```python
from build123d import *

# Parameters (mm, degrees)
EXTRUDE002_DEPTH = 2.15
SKETCH002_W      = 82.25
SKETCH002_H      = 45.1
SKETCH002_R      = 1.65
EXTRUDE003_DEPTH = 1.6
SKETCH004_W      = 7
SKETCH004_H      = 24
EXTRUDE004_DEPTH = 8.5
SKETCH048_W      = 9
SKETCH048_H      = 4
SKETCH048_W_2    = 4
SKETCH048_H_2    = 7.5
EXTRUDE049_DEPTH = 8.5
SKETCH005_W      = 7
SKETCH005_H      = 37.5
EXTRUDE005_DEPTH = 8.5


with BuildPart() as obj1:
    # Sketch003 → Extrude002 (new body)
    with BuildSketch(Plane.XY):
        Polygon((76.75, 36.6), (76.75, 17.05), (59.85, 17.05), (59.85, 6.1), (8.6, 6.1), (8.6, 39.3), (16.6, 39.3), (16.6, 36.6), align=None)
    extrude(amount=-EXTRUDE002_DEPTH)


with BuildPart() as obj2:
    # Sketch002 → Extrude003 (new body)
    with BuildSketch(Plane.XY):
        with Locations((41.125, 22.55)):
            Rectangle(SKETCH002_W, SKETCH002_H)
        with Locations((3, 42.1)):
            Circle(SKETCH002_R, mode=Mode.SUBTRACT)
        with Locations((79.25, 42.1)):
            Circle(SKETCH002_R, mode=Mode.SUBTRACT)
        with Locations((3, 3)):
            Circle(SKETCH002_R, mode=Mode.SUBTRACT)
        with Locations((79.25, 3)):
            Circle(SKETCH002_R, mode=Mode.SUBTRACT)
    extrude(amount=EXTRUDE003_DEPTH)


with BuildPart() as obj3:
    # Sketch004 → Extrude004 (new body)
    with BuildSketch(Plane.XY):
        with Locations((74.85, 25.84)):
            Rectangle(SKETCH004_W, SKETCH004_H)
    extrude(amount=EXTRUDE004_DEPTH)


with BuildPart() as obj3_1:
    # Extrude004 placement: moved
    add(obj3.part.moved(Location((0, 0, 1.6))))


with BuildPart() as obj4:
    # Sketch048 → Extrude049 (new body)
    with BuildSketch(Plane.XY):
        with Locations((47.75, 36.6)):
            Rectangle(SKETCH048_W, SKETCH048_H)
        with Locations((36.25, 21.85)):
            Rectangle(SKETCH048_W_2, SKETCH048_H_2)
    extrude(amount=EXTRUDE049_DEPTH)


with BuildPart() as obj5:
    # Sketch005 → Extrude005 (new body)
    with BuildSketch(Plane.XY):
        with Locations((9.77, 21.95)):
            Rectangle(SKETCH005_W, SKETCH005_H)
    extrude(amount=EXTRUDE005_DEPTH)


with BuildPart() as obj5_1:
    # Extrude005 placement: moved
    add(obj5.part.moved(Location((0, 0, 1.6))))

    # Fusion001: union obj1, obj2, obj3, obj4
    add(obj1.part)
    add(obj2.part)
    add(obj3_1.part)
    add(obj4.part)


with BuildPart() as obj5_2:
    # Fusion001 placement: moved
    add(obj5_1.part.moved(Location((0, 0, 4))))


solid = obj5_2.part
```
The listing builds one solid part. Answer for the finished solid, in the listing's coordinates (mm). A direction names the side the tool comes from. Coordinates: 2 decimals unless noted, no trailing zeros. Loops run counter-clockwise (first coordinate to the right, second up) from the corner with the lowest first, then second, coordinate; pieces in that order, holes last. Notation, with made-up numbers: (46, 9.25) - (66, 9.25) arc R25 cw to (66, 41.25) - close; hole circle Ø8 at (-15.75, 54.5). An arc over 180 degrees is marked (long way). Use a Markdown table: item, result. Add a question column.
1) The part is cut by section B-B, the plane y = 42.1. Give the vertices of the cut face in (x, z).
2) The part is cut by section D-D, the plane y = 11. Give the vertices of the cut face in (x, z), and give its area (3 significant figures).
3) The part is cut by section C-C, the plane z = 10.25. Give the vertices of the cut face in (x, y), and give its area (4 significant figures).
4) For faces 1 (the flat face through (75, 13.84, 10)), 2 (the flat face through (71.35, 26, 10)), 3 (the flat face through (8.6, 22, 3)), determine the directions among +Z, -Z, +X, -X, +Y, -Y from which every point of the face is accessible in a straight line to the end or side of a thin tool.
5) Given pin 1 (3.5 mm diameter, centred on x = 74.5, z = 9, fed in from +Y); pin 2 (2.5 mm diameter, centred on y = 20.5, z = 11, fed in from -X); pin 3 (2.5 mm diameter, centred on x = 79.25, y = 42.1, fed in from -Z); pin 4 (1.7 mm diameter, centred on x = 12, z = 2.5, fed in from +Y), each flat-ended and moving along its own axis, determine where each tip first touches the part or whether it passes through.
6) Find the intervals of material crossed by line 1 (X direction, y = 23, z = 8.25); line 2 (Y direction, x = 79.25, z = 4.55); line 3 (X direction, y = 28.5, z = 8), in increasing order.
7) The part is cut by section A-A, the plane x = 79.25. Give the vertices of the cut face in (y, z), and give its area (3 significant figures).
Here are the results:
| question | item | result |
|---|---|---|
| 1 | outline | (0, 4) - (1.35, 4) - (1.35, 5.6) - (0, 5.6) - close; (4.65, 4) - (77.6, 4) - (77.6, 5.6) - (4.65, 5.6) - close; (80.9, 4) - (82.25, 4) - (82.25, 5.6) - (80.9, 5.6) - close |
| 2 | outline | (0, 4) - (8.6, 4) - (8.6, 1.85) - (59.85, 1.85) - (59.85, 4) - (82.25, 4) - (82.25, 5.6) - (13.27, 5.6) - (13.27, 14.1) - (6.27, 14.1) - (6.27, 5.6) - (0, 5.6) - close |
| 2 | area | 301 mm^2 |
| 3 | outline | (6.27, 3.2) - (13.27, 3.2) - (13.27, 40.7) - (6.27, 40.7) - close; (34.25, 18.1) - (38.25, 18.1) - (38.25, 25.6) - (34.25, 25.6) - close; (43.25, 34.6) - (52.25, 34.6) - (52.25, 38.6) - (43.25, 38.6) - close; (71.35, 13.84) - (78.35, 13.84) - (78.35, 37.84) - (71.35, 37.84) - close |
| 3 | area | 496.5 mm^2 |
| 4 | face 1 | +Z, +X, -Y |
| 4 | face 2 | +Z, +Y, -Y |
| 4 | face 3 | -Z, -X, +Y, -Y |
| 5 | pin 1 | stops at y = 37.84 |
| 5 | pin 2 | stops at x = 6.27 |
| 5 | pin 3 | passes through |
| 5 | pin 4 | stops at y = 39.3 |
| 6 | line 1 | x = 6.27 to 13.27, 34.25 to 38.25, 71.35 to 78.35 |
| 6 | line 2 | y = 0 to 1.35, 4.65 to 40.45, 43.75 to 45.1 |
| 6 | line 3 | x = 6.27 to 13.27, 71.35 to 78.35 |
| 7 | outline | (0, 4) - (1.35, 4) - (1.35, 5.6) - (0, 5.6) - close; (4.65, 4) - (40.45, 4) - (40.45, 5.6) - (4.65, 5.6) - close; (43.75, 4) - (45.1, 4) - (45.1, 5.6) - (43.75, 5.6) - close |
| 7 | area | 61.6 mm^2 |
